Check sheet for the modelled part. Datum: model origin and axes. Units: mm. A direction names the side the tool comes from. Round coordinates to 2 decimals unless told otherwise and drop trailing zeros. Order: outer loops, then holes, each group sorted by start corner. A loop starts at its lowest first (then second) coordinate and runs counter-clockwise, first axis right, second up. Notation, with made-up numbers: (-24, 12) -> (14, 12) arc R22 cw to (14, 41) -> close; hole circle Ø5 at (-12, 29). An arc over 180 degrees is marked (long way). Use CSV: the item, a comma, the result in double quotes.
```python
from build123d import *

# Parameters (mm, degrees)
FILLET1_R          = 10
FILLET2_R          = 10
FILLET3_R          = 10
FILLET4_R          = 10
SKETCH3_R          = 7.5
CUT_EXTRUDE1_DEPTH = 73.284161495


with BuildPart() as part:
    # Sketch2 → Revolve1 (revolve)
    with BuildSketch(Plane(origin=(0, 0, 0), x_dir=(0, 0, -1), z_dir=(1, 0, 0))):
        with BuildLine():
            Line((0, 7.5), (-31, 7.5))
            Line((-31, 7.5), (-31, 6.5))
            Line((-31, 6.5), (-35, 6.5))
            Line((-35, 6.5), (-35, 7.5))
            Line((-35, 7.5), (-50, 7.5))
            Line((-50, 7.5), (-50, 5.5))
            ThreePointArc((-50, 5.5), (-46.147650045, 0), (-50, -5.5))
            Line((-50, -5.5), (-50, -7.5))
            Line((-50, -7.5), (-35, -7.5))
            Line((-35, -7.5), (-35, -6.5))
            Line((-35, -6.5), (-31, -6.5))
            Line((-31, -6.5), (-31, -7.5))
            Line((-31, -7.5), (0, -7.5))
            Line((0, -7.5), (0, 7.5))
        make_face()
    revolve(axis=Axis((0, 55.434917487, 0), (0, -1, 0)))

    # Fillet1
    # the kernel refuses this fillet: 10 mm, written as the material it takes off along each edge
    with BuildSketch(Plane(origin=(0, 7.5, 0), x_dir=(0, 0, 1), z_dir=(1, 0, 0))) as fillet1_piece_1:
        with BuildLine():
            CenterArc((39.358898944, 10), FILLET1_R, 244.158067237, 25.841932763)
            Line((39.358898944, 0), (39.358898944, -0.2))
            Line((39.358898944, -0.2), (35, -0.2))
            Line((35, -0.2), (34.8, 0))
            ThreePointArc((34.8, 0), (34.8, 0.5), (34.912822021, 0.82))
            Line((34.912822021, 0.82), (35, 1))
        make_face()
    revolve(axis=Axis((0, 7.5, 0), (0, -1, 0)), mode=Mode.SUBTRACT)

    # Fillet2
    # the kernel refuses this fillet: 10 mm, written as the material it takes off along each edge
    with BuildSketch(Plane(origin=(0, 7.5, 0), x_dir=(0, 0, 1), z_dir=(1, 0, 0))) as fillet2_piece_1:
        with BuildLine():
            CenterArc((26.641101056, 10), FILLET2_R, 270, 25.841932763)
            Line((26.641101056, 0), (26.641101056, -0.2))
            Line((26.641101056, -0.2), (31, -0.2))
            Line((31, -0.2), (31.2, 0))
            ThreePointArc((31.2, 0), (31.2, 0.5), (31.087177979, 0.82))
            Line((31.087177979, 0.82), (31, 1))
        make_face()
    revolve(axis=Axis((0, 7.5, 0), (0, -1, 0)), mode=Mode.SUBTRACT)

    # Fillet3
    # the kernel refuses this fillet: 10 mm, written as the material it takes off along each edge
    with BuildSketch(Plane(origin=(0, -7.5, 0), x_dir=(0, 0, 1), z_dir=(1, 0, 0))) as fillet3_piece_1:
        with BuildLine():
            CenterArc((39.358898944, -10), FILLET3_R, 90, 25.841932763)
            Line((35, -1), (34.912822021, -0.82))
            ThreePointArc((34.912822021, -0.82), (34.8, -0.5), (34.8, 0))
            Line((34.8, 0), (35, 0.2))
            Line((35, 0.2), (39.358898944, 0.2))
            Line((39.358898944, 0.2), (39.358898944, 0))
        make_face()
    revolve(axis=Axis((0, -7.5, 0), (0, -1, 0)), mode=Mode.SUBTRACT)

    # Fillet4
    # the kernel refuses this fillet: 10 mm, written as the material it takes off along each edge
    with BuildSketch(Plane(origin=(0, -7.5, 0), x_dir=(0, 0, 1), z_dir=(1, 0, 0))) as fillet4_piece_1:
        with BuildLine():
            CenterArc((26.641101056, -10), FILLET4_R, 64.158067237, 25.841932763)
            Line((26.641101056, 0), (26.641101056, 0.2))
            Line((26.641101056, 0.2), (31, 0.2))
            Line((31, 0.2), (31.2, 0))
            ThreePointArc((31.2, 0), (31.2, -0.5), (31.087177979, -0.82))
            Line((31.087177979, -0.82), (31, -1))
        make_face()
    revolve(axis=Axis((0, -7.5, 0), (0, -1, 0)), mode=Mode.SUBTRACT)

    # Sketch3 → Cut-Extrude1 (cut, through all)
    with BuildSketch(Plane.XZ.offset(7.5)):
        with Locations(Location((0, 0, 0), (0, 0, 270))):
            Circle(SKETCH3_R)
    extrude(amount=-CUT_EXTRUDE1_DEPTH, mode=Mode.SUBTRACT)


solid = part.part
```
Q1. Mould release check, pull along X, two halves, no side actions. Record for faces 1 (the face through (-15.02, -6.51, 47.69)), 2 (the face through (23.2, -6.5, -20.9)), 3 (the face through (6, -7.5, 6)): pulls with the +X half, pulls with the -X half, needs draft (parallel to the pull), parting line crosses it, or undercut.
Result sheet:
face 1,"parting line crosses it"
face 2,"undercut"
face 3,"needs draft"
Q2. Access from +Z, -Z, +X, -X, +Y, -Y to the whole of each face (thin tool, end or side, straight path). Record for faces 4 (the face through (23.2, 6.5, 20.9)), 5 (the face through (37, 7.5, -15)).
Result sheet:
face 4,"+Y"
face 5,"+Z, -Z, +X, -X, +Y"
Q3. Sectioned sample at B-B, the plane z = 0. Enter the section's corners in (x, y).
Result sheet:
outline,"(-50, -7.5) -> (-39.36, -7.5) arc R10 ccw to (-35, -6.5) -> (-31, -6.5) arc R10 ccw to (-26.64, -7.5) -> (-7.5, -7.5) -> (-7.5, 7.5) -> (-26.64, 7.5) arc R10 ccw to (-31, 6.5) -> (-35, 6.5) arc R10 ccw to (-39.36, 7.5) -> (-50, 7.5) -> (-50, 5.5) arc R5.85 cw to (-50, -5.5) -> close; (7.5, -7.5) -> (26.64, -7.5) arc R10 ccw to (31, -6.5) -> (35, -6.5) arc R10 ccw to (39.36, -7.5) -> (50, -7.5) -> (50, -5.5) arc R5.85 cw to (50, 5.5) -> (50, 7.5) -> (39.36, 7.5) arc R10 ccw to (35, 6.5) -> (31, 6.5) arc R10 ccw to (26.64, 7.5) -> (7.5, 7.5) -> close"
Q4. Scan lines: L1, parallel to X at y = -2.5, z = 0; L2, parallel to X at y = 2.75, z = 0; L3, parallel to Z at x = 4, y = -3.5. Record each from-to range of solid material in increasing order.
Result sheet:
L1,"x = -46.71 to -7.5, 7.5 to 46.71"
L2,"x = -46.83 to -7.5, 7.5 to 46.83"
L3,"z = -47.14 to -6.34, 6.34 to 47.14"
Q5. Go/stop test with flat-tipped pins: pin 1 (2 mm diameter, centred on y = -5.5, z = 32.5, fed in from +X); pin 2 (1 mm diameter, centred on x = -29.5, y = -0.5, fed in from +Z); pin 3 (1 mm diameter, centred on x = -1, y = -3, fed in from -Z); pin 4 (12 mm diameter, centred on x = 0, z = 0, fed in from -Y). Record where each tip stops, or that it passes through.
Result sheet:
pin 1,"stops at x = 38.83"
pin 2,"stops at z = 35.93"
pin 3,"stops at z = -47.3"
pin 4,"passes through"
Q6. Sectioned sample at A-A, the plane x = 0. Enter the section's corners in (y, z), then the cut area to 3 significant figures.
Result sheet:
outline,"(-7.5, -50) -> (-5.5, -50) arc R5.85 cw to (5.5, -50) -> (7.5, -50) -> (7.5, -39.36) arc R10 ccw to (6.5, -35) -> (6.5, -31) arc R10 ccw to (7.5, -26.64) -> (7.5, -7.5) -> (-7.5, -7.5) -> (-7.5, -26.64) arc R10 ccw to (-6.5, -31) -> (-6.5, -35) arc R10 ccw to (-7.5, -39.36) -> close; (-7.5, 7.5) -> (7.5, 7.5) -> (7.5, 26.64) arc R10 ccw to (6.5, 31) -> (6.5, 35) arc R10 ccw to (7.5, 39.36) -> (7.5, 50) -> (5.5, 50) arc R5.85 cw to (-5.5, 50) -> (-7.5, 50) -> (-7.5, 39.36) arc R10 ccw to (-6.5, 35) -> (-6.5, 31) arc R10 ccw to (-7.5, 26.64) -> close"
area,"1,190 mm^2"
Q7. Sectioned sample at C-C, the plane y = -0.75. Enter the section's corners in (x, z), then the cut area to 3 significant figures.
Result sheet:
outline,"circle Ø92.39 at (0, 0); hole circle Ø15 at (0, 0)"
area,"6,530 mm^2"
